from build123d import *

# Parameters (mm, degrees)
BOSS_EXTRUDE4_DEPTH = 10
SKETCH6_W           = 46.8
SKETCH6_H           = 26.2
SKETCH6_W_2         = 40.8
SKETCH6_H_2         = 20.2
BOSS_EXTRUDE5_DEPTH = 28
SKETCH8_W           = 8.35
SKETCH8_H           = 20
CUT_EXTRUDE2_DEPTH  = 28
SKETCH12_W          = 26.2
SKETCH12_H          = 28
BOSS_EXTRUDE6_DEPTH = 7
SKETCH13_W          = 8.35
SKETCH13_H          = 4.5
SKETCH13_H_2        = 3.5
BOSS_EXTRUDE7_DEPTH = 7


with BuildPart() as part:
    # Sketch2 → Boss-Extrude4 (new body)
    with BuildSketch(Plane(origin=(0, 0, 0), x_dir=(1, 0, 0), z_dir=(0, 1, 0))):
        with BuildLine():
            Line((-74.999999302, 50.000000465), (75.000000698, 50.000000465))
            ThreePointArc((75.000000698, 50.000000465), (124.999999302, -9.31e-07), (74.999997905, -49.999999535))
            Line((74.999997905, -49.999999535), (-74.999999302, -49.999999535))
            Line((-74.999999302, -49.999999535), (-74.999999302, 50.000000465))
        make_face()
    extrude(amount=BOSS_EXTRUDE4_DEPTH)

    # Sketch6 → Boss-Extrude5 (add)
    with BuildSketch(Plane(origin=(0, 10, 0), x_dir=(1, 0, 0), z_dir=(0, 1, 0))):
        with Locations((74.999999302, 4.65e-07)):
            Rectangle(SKETCH6_W, SKETCH6_H)
        with Locations((74.999999302, 4.65e-07)):
            Rectangle(SKETCH6_W_2, SKETCH6_H_2, mode=Mode.SUBTRACT)
    extrude(amount=BOSS_EXTRUDE5_DEPTH)

    # Sketch8 → Cut-Extrude2 (cut)
    with BuildSketch(Plane.ZY.offset(-51.599999302)):
        with Locations((-4.65e-07, 23.5)):
            Rectangle(SKETCH8_W, SKETCH8_H)
    extrude(amount=-CUT_EXTRUDE2_DEPTH, mode=Mode.SUBTRACT)

    # Sketch12 → Boss-Extrude6 (add)
    with BuildSketch(Plane(origin=(98.399999302, 0, 0), x_dir=(0, 0, -1), z_dir=(1, 0, 0))):
        with Locations((4.65e-07, 24)):
            Rectangle(SKETCH12_W, SKETCH12_H)
    extrude(amount=BOSS_EXTRUDE6_DEPTH)

    # Sketch13 → Boss-Extrude7 (add)
    with BuildSketch(Plane.ZY.offset(-51.599999302)):
        Polygon((-4.175000465, 10), (-4.175000465, 13.5), (-4.175000465, 33.5), (-4.175000465, 38), (-13.100000465, 38), (-13.100000465, 10), align=None)
        with Locations((-4.65e-07, 35.75)):
            Rectangle(SKETCH13_W, SKETCH13_H)
        Polygon((4.174999535, 33.5), (4.174999535, 13.5), (4.174999535, 10), (13.099999535, 10), (13.099999535, 38), (4.174999535, 38), align=None)
        with Locations((-4.65e-07, 11.75)):
            Rectangle(SKETCH13_W, SKETCH13_H_2)
    extrude(amount=BOSS_EXTRUDE7_DEPTH)


solid = part.part
Here's how the part is built. I have some questions about the finished solid (model axes, mm). A direction names the side the tool comes from. Coordinates: 2 decimals unless noted, no trailing zeros. Loops run counter-clockwise (first coordinate to the right, second up) from the corner with the lowest first, then second, coordinate; pieces in that order, holes last. Notation, with made-up numbers: (-6, -7) -> (21, -7) arc R20 ccw to (21, 14) -> close; hole circle Ø1 at (55, 48.5). An arc over 180 degrees is marked (long way). Use one line per item in the form item = value. Start each with the question number.
(1) If we section it at C-C (y = 20): Please give me the cut outline in (x, z) (3 decimals), then the cut area to 3 significant figures.
(2) On a 3-axis mill with a long thin cutter (end or side, diameter ignored), from which of +Z, -Z, +X, -X, +Y, -Y can I reach the whole of each face in a straight line? I mean faces 1 (the face through (50, 23, -4.175)), 2 (the face through (75, 24, 10.1)), 3 (the face through (44.6, 24, -6)). Say none if no direction works.
(3) If we section it at A-A (z = 0): Please give me the cut outline in (x, y), then the cut area to 3 significant figures.
(4) If we section it at B-B (x = 49): Please give me the cut outline in (y, z) (3 decimals).
(5) We'd pull the mould along Y, two halves only. Please class faces 4 (the face through (50, 33.5, 0)), 5 (the face through (75, 10, 0)), 6 (the face through (105.4, 24, 0)): pulls with the +Y half, pulls with the -Y half, needs draft (parallel to the pull), parting line crosses it, or undercut.
(6) Will these pins go through, and if not, where does the flat tip stop? pin 1 (2 mm diameter, centred on y = 22.5, z = -6, fed in from -X); pin 2 (8 mm diameter, centred on y = 29, z = 20.5, fed in from -X); pin 3 (8 mm diameter, centred on y = 20, z = 6.5, fed in from +X); pin 4 (16 mm diameter, centred on x = 72.5, z = 0, fed in from +Y).
(7) If we section it at D-D (z = -23): Please give me the cut outline in (x, y).
(8) Please list where these lines run through material, in increasing order: line 1 along X through (y, z) = (36, -6); line 2 along Z through (x, y) = (68, 28.5); line 3 along X through (y, z) = (19.5, -11).
Verdict:
q1.outline = (44.6, -13.1) -> (105.4, -13.1) -> (105.4, 13.1) -> (44.6, 13.1) -> (44.6, 4.175) -> (54.6, 4.175) -> (54.6, 10.1) -> (95.4, 10.1) -> (95.4, -10.1) -> (54.6, -10.1) -> (54.6, -4.175) -> (44.6, -4.175) -> close
q1.area = 685 mm²
q2.face_1 = -X
q2.face_2 = +Y
q2.face_3 = +Z, -Z, -X, +Y
q3.outline = (-75, 0) -> (125, 0) -> (125, 10) -> (105.4, 10) -> (105.4, 38) -> (95.4, 38) -> (95.4, 10) -> (54.6, 10) -> (54.6, 13.5) -> (44.6, 13.5) -> (44.6, 10) -> (-75, 10) -> close; (44.6, 33.5) -> (54.6, 33.5) -> (54.6, 38) -> (44.6, 38) -> close
q3.area = 2,360 mm²
q4.outline = (0, -50) -> (10, -50) -> (10, -13.1) -> (38, -13.1) -> (38, 13.1) -> (10, 13.1) -> (10, 50) -> (0, 50) -> close; hole (13.5, -4.175) -> (33.5, -4.175) -> (33.5, 4.175) -> (13.5, 4.175) -> close
q5.face_4 = undercut
q5.face_5 = pulls with the +Y half
q5.face_6 = needs draft
q6.pin_1 = 44.6
q6.pin_2 = through
q6.pin_3 = 105.4
q6.pin_4 = 10
q7.outline = (-75, 0) -> (119.4, 0) -> (119.4, 10) -> (-75, 10) -> close
q8.line_1 = 44.6 to 54.6, 95.4 to 105.4
q8.line_2 = -13.1 to -10.1, 10.1 to 13.1
q8.line_3 = 44.6 to 105.4
